Geometry check sheet. Reference: the model listing, model coordinates, mm. Face numbers are marked on the shaded views. A direction names the side the tool comes from. Coordinates: 2 decimals unless noted, no trailing zeros. Loops run counter-clockwise (first coordinate to the right, second up) from the corner with the lowest first, then second, coordinate; pieces in that order, holes last.
from build123d import *

# Parameters (mm, degrees)
SKETCH_1_W             = 426
SKETCH_1_H             = 40.7
SM_BASE_FLANGE_1_DEPTH = 1.5
SM_EDGE_FLANGE_2_DEPTH = 40.7
SM_EDGE_FLANGE_3_DEPTH = 426
SM_EDGE_FLANGE_4_DEPTH = 40.7


# Sheet-metal steps are written as plain solids
with BuildPart() as part:
    # Sketch 1 → Базовая кромка1 (new body)
    with BuildSketch(Plane.XY):
        with Locations((213, 20.35)):
            Rectangle(SKETCH_1_W, SKETCH_1_H)
    extrude(amount=-SM_BASE_FLANGE_1_DEPTH)

    # Ребро-кромка2 section (across the edge) → Ребро-кромка2 (add)
    with BuildSketch(Plane(origin=(-1.5, 0, -1.5), x_dir=(1, 0, 0), z_dir=(0, 1, 0))):
        with BuildLine():
            Line((-1.5, 1.5), (-1.5, 13.5))
            Line((-1.5, 13.5), (0, 13.5))
            Line((0, 13.5), (0, 1.5))
            ThreePointArc((0, 1.5), (0.439339828, 0.439339828), (1.5, 0))
            Line((1.5, 0), (1.5, -1.5))
            ThreePointArc((1.5, -1.5), (-0.621320344, -0.621320344), (-1.5, 1.5))
        make_face()
    extrude(amount=SM_EDGE_FLANGE_2_DEPTH)

    # Ребро-кромка3 section (across the edge) → Ребро-кромка3 (add)
    with BuildSketch(Plane(origin=(426, -1.5, -1.5), x_dir=(0, 1, 0), z_dir=(-1, 0, 0))):
        with BuildLine():
            Line((-1.5, 1.5), (-1.5, 13.5))
            Line((-1.5, 13.5), (0, 13.5))
            Line((0, 13.5), (0, 1.5))
            ThreePointArc((0, 1.5), (0.439339828, 0.439339828), (1.5, 0))
            Line((1.5, 0), (1.5, -1.5))
            ThreePointArc((1.5, -1.5), (-0.621320344, -0.621320344), (-1.5, 1.5))
        make_face()
    extrude(amount=SM_EDGE_FLANGE_3_DEPTH)

    # Ребро-кромка4 section (across the edge) → Ребро-кромка4 (add)
    with BuildSketch(Plane(origin=(427.5, 40.7, -1.5), x_dir=(-1, 0, 0), z_dir=(0, -1, 0))):
        with BuildLine():
            Line((-1.5, 1.5), (-1.5, 13.5))
            Line((-1.5, 13.5), (0, 13.5))
            Line((0, 13.5), (0, 1.5))
            ThreePointArc((0, 1.5), (0.439339828, 0.439339828), (1.5, 0))
            Line((1.5, 0), (1.5, -1.5))
            ThreePointArc((1.5, -1.5), (-0.621320344, -0.621320344), (-1.5, 1.5))
        make_face()
    extrude(amount=SM_EDGE_FLANGE_4_DEPTH)


solid = part.part
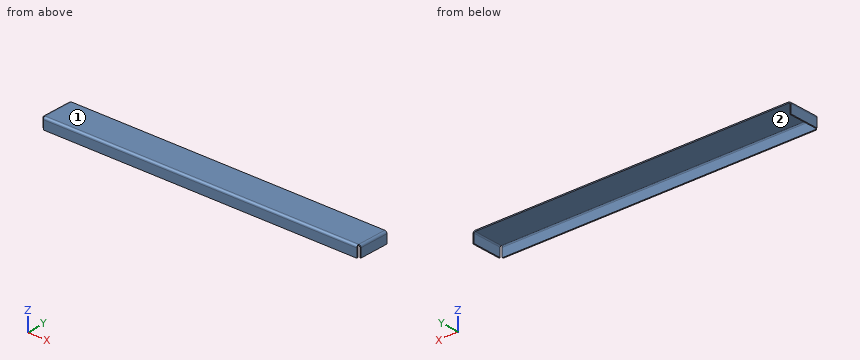
1) Section check C-C on x = 354.5. Record the cut outline in (y, z).
Data:
outline: (-3, -15) - (-1.5, -15) - (-1.5, -3) arc R1.5 cw to (0, -1.5) - (40.7, -1.5) - (40.7, 0) - (0, 0) arc R3 ccw to (-3, -3) - close
2) Material ranges on probe 1 along X at (y, z) = (2.5, -13.5); probe 2 along Z at (x, y) = (25, 10); probe 3 along Y at (x, z) = (20.5, -4.75), recorded low to high.
Data:
probe 1: x = -3 to -1.5, 427.5 to 429
probe 2: z = -1.5 to 0
probe 3: y = -3 to -1.5
3) Section check A-A on z = -12.5. Record the cut outline in (x, y), and give its area (3 significant figures).
Data:
outline: (-3, 0) - (-1.5, 0) - (-1.5, 40.7) - (-3, 40.7) - close; (0, -3) - (426, -3) - (426, -1.5) - (0, -1.5) - close; (427.5, 0) - (429, 0) - (429, 40.7) - (427.5, 40.7) - close
area: 761 mm2
4) Section check B-B on y = 31. Record the cut outline in (x, z).
Data:
outline: (-3, -15) - (-1.5, -15) - (-1.5, -3) arc R1.5 cw to (0, -1.5) - (426, -1.5) arc R1.5 cw to (427.5, -3) - (427.5, -15) - (429, -15) - (429, -3) arc R3 ccw to (426, 0) - (0, 0) arc R3 ccw to (-3, -3) - close
5) Depth check by flat-ended pin: pin 1 (8 mm diameter, centred on x = 60, z = -9, fed in from +Y); pin 2 (0.9 mm diameter, centred on x = -1.5, z = -4, fed in from -Y); pin 3 (1 mm diameter, centred on x = 100, y = 8.5, fed in from -Z); pin 4 (0.9 mm diameter, centred on y = -1, z = -10, fed in from +X). Enter the tip coordinate at first touch or a pass-through.
Data:
pin 1: stops at y = -1.5
pin 2: stops at y = 0
pin 3: stops at z = -1.5
pin 4: passes through
6) Access from +Z, -Z, +X, -X, +Y, -Y to the whole of each face (thin tool, end or side, straight path). Record for the marked faces 1 and 2.
Data:
face 1: +Z, +X, -X, +Y, -Y
face 2: -Z, +Y
